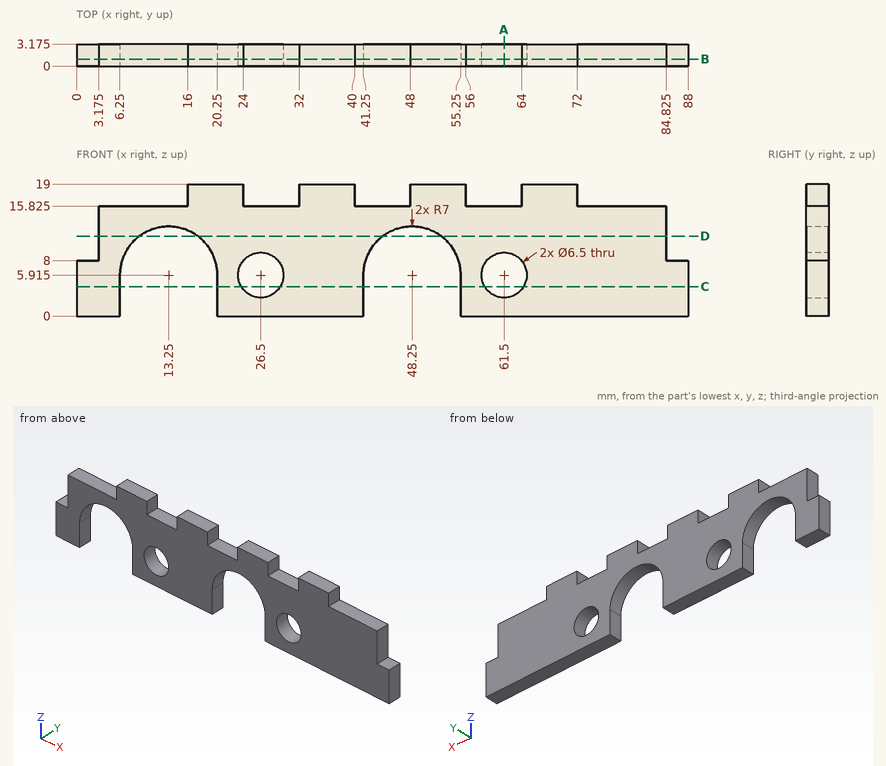
The figure shows three views and two pictorial views of one solid part (mm, origin at its lowest corner). Answer the questions. Coordinates: 2 decimals unless noted, no trailing zeros. Loops run counter-clockwise (first coordinate to the right, second up) from the corner with the lowest first, then second, coordinate; pieces in that order, holes last. Notation, with made-up numbers: (-12.5, -14.5) - (14.5, -14.5) arc R16 cw to (14.5, 5.5) - close; hole circle Ø3 at (68, 7.5). An arc over 180 degrees is marked (long way). Answer in a Markdown table with one row per item.
Q1. Straight lines are drawn through the part: line 1 along X through (y, z) = (0.9, 5.75); line 2 along X through (y, z) = (1.75, 16); line 3 along X through (y, z) = (1.1, 1.25). For each, find the intervals that lie inside material, in ascending order. Write a range as [from, to].
Here are the results:
| item | result |
|---|---|
| line 1 | x = [0, 6.25], [20.25, 23.25], [29.75, 41.25], [55.25, 58.25], [64.75, 88] |
| line 2 | x = [16, 24], [32, 40], [48, 56], [64, 72] |
| line 3 | x = [0, 6.25], [20.25, 41.25], [55.25, 88] |
Q2. Find section B-B on y = 1. Count the separate pieces of the cut face and the enclosed holes in it, plus the area to 3 significant figures.
Here are the results:
| item | result |
|---|---|
| separate pieces | 1 |
| enclosed holes | 2 |
| area | 1,060 mm^2 |
Q3. Find section A-A on x = 61.5. Write down the section's boundary in (y, z) (3 decimals).
Here are the results:
| item | result |
|---|---|
| outline | (0, 0) - (3.175, 0) - (3.175, 2.665) - (0, 2.665) - close; (0, 9.165) - (3.175, 9.165) - (3.175, 15.825) - (0, 15.825) - close |
Q4. Find section C-C on z = 4.25. Write down the section's boundary in (x, y) (3 decimals).
Here are the results:
| item | result |
|---|---|
| outline | (0, 0) - (6.25, 0) - (6.25, 3.175) - (0, 3.175) - close; (20.25, 0) - (23.709, 0) - (23.709, 3.175) - (20.25, 3.175) - close; (29.291, 0) - (41.25, 0) - (41.25, 3.175) - (29.291, 3.175) - close; (55.25, 0) - (58.709, 0) - (58.709, 3.175) - (55.25, 3.175) - close; (64.291, 0) - (88, 0) - (88, 3.175) - (64.291, 3.175) - close |
Q5. Find section D-D on z = 11.5. Write down the section's boundary in (x, y) (3 decimals).
Here are the results:
| item | result |
|---|---|
| outline | (3.175, 0) - (9.03, 0) - (9.03, 3.175) - (3.175, 3.175) - close; (17.47, 0) - (44.03, 0) - (44.03, 3.175) - (17.47, 3.175) - close; (52.47, 0) - (84.825, 0) - (84.825, 3.175) - (52.47, 3.175) - close |
Q6. Given P1, Ø8, axis at x = 26, z = 9.5, coming from the -Y side; P2, Ø1.6, axis at y = 2, z = 18, coming from the +X side; P3, Ø1.6, axis at y = 1, z = 17, coming from the -X side; P4, Ø1.6, axis at x = 86.5, y = 1.5, coming from the +Z side, each flat-ended and moving along its own axis, determine where each tip first touches the part or whether it passes through.
Here are the results:
| item | result |
|---|---|
| P1 | stops at y = 0 |
| P2 | stops at x = 72 |
| P3 | stops at x = 16 |
| P4 | stops at z = 8 |
